Build history of the part. All positions in model axes, mm. A direction names the side the tool comes from. Round coordinates to 2 decimals unless told otherwise and drop trailing zeros. Loops run counter-clockwise (first coordinate to the right, second up) from the corner with the lowest first, then second, coordinate; pieces in that order, holes last.
from build123d import *

# Parameters (mm, degrees)
F1_DEPTH = 6.5
F2_W     = 8
F2_H     = 8
F3_DEPTH = 2
F4_R     = 1.5
F5_DEPTH = 25


with BuildPart() as f1:
    # F0 (on Front) → F1 (new body, symmetric)
    with BuildSketch(Plane.XZ):
        with BuildLine():
            Line((3, 0), (5, 0))
            ThreePointArc((5, 0), (0, 5), (-5, 0))
            Line((-5, 0), (-3, 0))
            ThreePointArc((-3, 0), (0, 3), (3, 0))
        make_face()
    extrude(amount=F1_DEPTH, both=True)

    # F2 (on Top) → F3 (join)
    with BuildSketch(Plane.XY):
        with Locations((-7, 0)):
            Rectangle(F2_W, F2_H)
    extrude(amount=F3_DEPTH)

    # F4 (on face) → F5 (cut)
    with BuildSketch(Plane.XY.offset(2)):
        with Locations((-8, 0)):
            Circle(F4_R)
    extrude(amount=-F5_DEPTH, mode=Mode.SUBTRACT)


solid = f1.part
(1) Slice it at A-A on x = -8. List the corners of the cut face in (y, z), plus the area to 3 significant figures.
Responses:
outline: (-4, 0) - (-1.5, 0) - (-1.5, 2) - (-4, 2) - close; (1.5, 0) - (4, 0) - (4, 2) - (1.5, 2) - close
area: 10.0 mm2
(2) Slice it at B-B on y = 0. List the corners of the cut face in (x, z).
Responses:
outline: (-11, 0) - (-9.5, 0) - (-9.5, 2) - (-11, 2) - close; (-6.5, 0) - (-3, 0) arc R3 cw to (3, 0) - (5, 0) arc R5 ccw to (-4.58, 2) - (-6.5, 2) - close
(3) Pin check, flat tips, straight feed: P1, Ø5, axis at x = -8.5, y = -1.5, coming from the +Z side; P2, Ø1, axis at x = -2, y = 2.5, coming from the +Z side; P3, Ø4, axis at x = 0.5, y = -4.5, coming from the -Z side. Stop position of each tip, or through.
Responses:
P1: stops at z = 2
P2: stops at z = 4.77
P3: stops at z = 1.66
(4) Pull direction X, two halves, no side cores. Call faces 3 (the face through (0, 0, 5)), 4 (the face through (4, 0, 0)), 5 (the face through (-9.5, 0.07, 1.01)), 6 (the face through (0, 0, 3)): +X half, -X half, draft (parallel to the pull), parting line (faces both ways), or undercut.
Responses:
face 3: parting line
face 4: draft
face 5: undercut
face 6: undercut
(5) Slice it at D-D on y = -3.5. List the corners of the cut face in (x, z), plus the area to 3 significant figures.
Responses:
outline: (-11, 0) - (-3, 0) arc R3 cw to (3, 0) - (5, 0) arc R5 ccw to (-4.58, 2) - (-11, 2) - close
area: 37.4 mm2
(6) Slice it at C-C on z = 1.2. List the corners of the cut face in (x, y).
Responses:
outline: (-11, -4) - (-4.85, -4) - (-4.85, -6.5) - (-2.75, -6.5) - (-2.75, 6.5) - (-4.85, 6.5) - (-4.85, 4) - (-11, 4) - close; (2.75, -6.5) - (4.85, -6.5) - (4.85, 6.5) - (2.75, 6.5) - close; hole circle Ø3 at (-8, 0)
(7) Probe line 1 (Y direction, x = -8, z = 0.5); line 2 (X direction, y = 0.5, z = 0.4); line 3 (X direction, y = 2.5, z = 2.7). List the from-to ranges inside material, lowest first.
Responses:
line 1: y = -4 to -1.5, 1.5 to 4
line 2: x = -11 to -9.41, -6.59 to -2.97, 2.97 to 4.98
line 3: x = -4.21 to -1.31, 1.31 to 4.21
(8) Which spindle directions (+Z, -Z, +X, -X, +Y, -Y) get a long thin tool onto all of the face, cutting with end or side? Do faces 1 (the face through (-6, 0, 2)), 2 (the face through (-11, 0, 1)). Say none if no direction does.
Responses:
face 1: +Z, -X, +Y, -Y
face 2: +Z, -Z, -X, +Y, -Y
